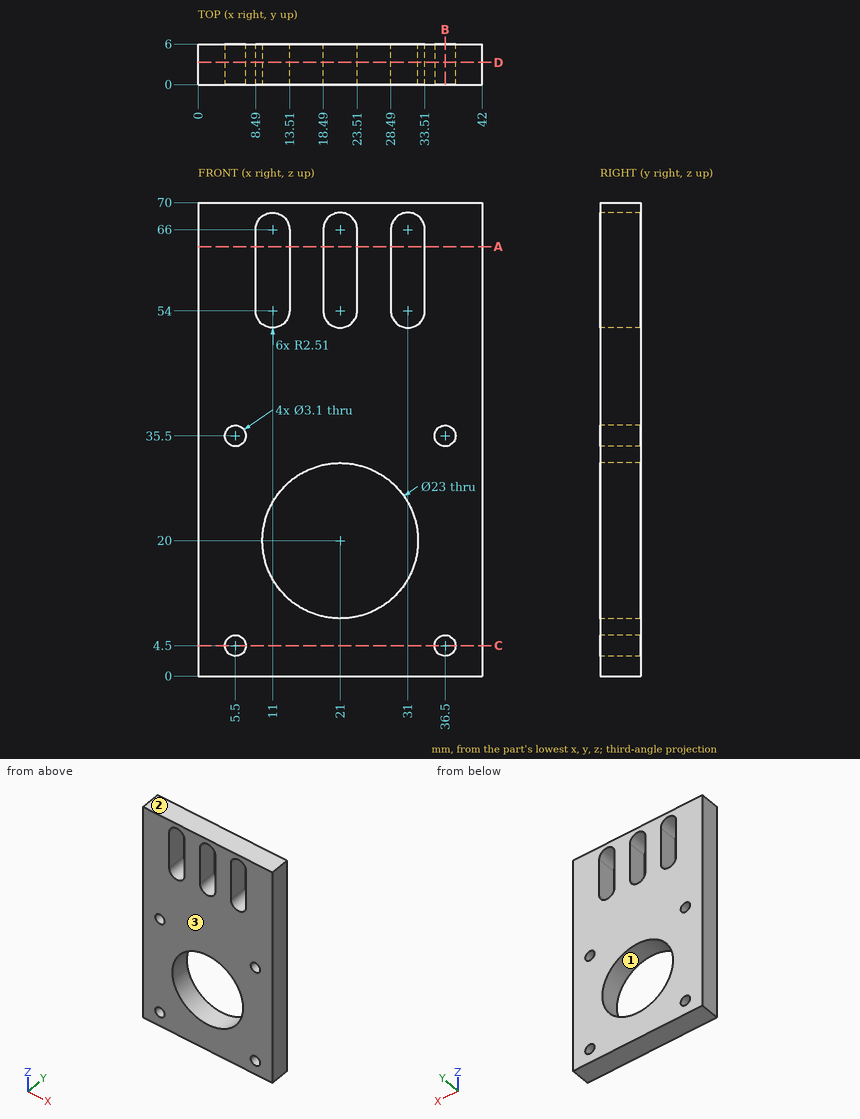
Source: three-view drawing plus pictorial views. Frame: mm from the lowest corner of the part. Round coordinates to 2 decimals unless told otherwise and drop trailing zeros. Order: outer loops, then holes, each group sorted by start corner. A loop starts at its lowest first (then second) coordinate and runs counter-clockwise, first axis right, second up. Notation, with made-up numbers: (-34, -21.5) - (22, -21.5) arc R12 ccw to (22, -11.5) - close; hole circle Ø9 at (-0.5, -11.75). An arc over 180 degrees is marked (long way). Write each question's results on one line, items separated by ' | '.
Item 1: Section C-C, the plane z = 4.5. Return the cut outline in (x, y).
Completed:
outline: (0, 0) - (3.95, 0) - (3.95, 6) - (0, 6) - close; (7.05, 0) - (34.95, 0) - (34.95, 6) - (7.05, 6) - close; (38.05, 0) - (42, 0) - (42, 6) - (38.05, 6) - close
Item 2: Material intervals for line 1 along Z through (x, y) = (36.5, 1.85); line 2 along X through (y, z) = (1.7, 4.5); line 3 along X through (y, z) = (2.8, 56), sorted ascending. Write a range as [from, to].
Completed:
line 1: [0, 2.95], [6.05, 33.95], [37.05, 70] | line 2: [0, 3.95], [7.05, 34.95], [38.05, 42] | line 3: [0, 8.49], [13.51, 18.49], [23.51, 28.49], [33.51, 42]
Item 3: Mould query, pull axis Z, two halves, no side actions, for the marked faces 1, 2 and 3. Classes: pulls with the +Z half, pulls with the -Z half, needs draft (parallel to the pull), parting line crosses it, or undercut.
Completed:
face 1: undercut | face 2: pulls with the +Z half | face 3: needs draft
Item 4: Section A-A, the plane z = 63.5. Return the cut outline in (x, y), and give its area (3 significant figures).
Completed:
outline: (0, 0) - (8.49, 0) - (8.49, 6) - (0, 6) - close; (13.51, 0) - (18.49, 0) - (18.49, 6) - (13.51, 6) - close; (23.51, 0) - (28.49, 0) - (28.49, 6) - (23.51, 6) - close; (33.51, 0) - (42, 0) - (42, 6) - (33.51, 6) - close | area: 162 mm^2
Item 5: Section D-D, the plane y = 3.3. State how many separate pieces and enclosed holes the cut face has, and give its area (3 significant figures).
Completed:
separate pieces: 1 | enclosed holes: 8 | area: 2,250 mm^2
Item 6: Section B-B, the plane x = 36.5. Return the cut outline in (y, z), and give its area (3 significant figures).
Completed:
outline: (0, 0) - (6, 0) - (6, 2.95) - (0, 2.95) - close; (0, 6.05) - (6, 6.05) - (6, 33.95) - (0, 33.95) - close; (0, 37.05) - (6, 37.05) - (6, 70) - (0, 70) - close | area: 383 mm^2
